Autodesk Inventor part; units mm, degrees
ref_plane "YZ Plane" through (0, 0, 0) normal (1, 0, 0) x (0, 1, 0)
ref_plane "XZ Plane" through (0, 0, 0) normal (0, 1, 0) x (-1, 0, 0)
ref_plane "XY Plane" through (0, 0, 0) normal (0, 0, 1) x (1, 0, 0)
sketch "Sketch1" plane through (0, 0, 0) normal (0, 0, 1) x (1, 0, 0)
  circle A0 centre (0, 0) radius 3.175
  circle A1 centre (0, 0) radius 3.9688
  dimension "d0" = 6.35
  dimension "d1" = 7.9375
extrude "Extrusion1" add sketch "Sketch1" along normal blind 1.8415 contours A0 | A1
extrude "Extrusion2" add sketch "Sketch1" against normal blind 6.35 contours A0
sketch "Sketch2" plane through (0, 0, 1.8415) normal (0, 0, 1) x (1, 0, 0)
  circle A0 centre (0, 0) radius 3.9687
  circle A1 centre (0, 0) radius 3.175
  dimension "d6" = 6.35
extrude "Extrusion3" add sketch "Sketch2" along normal blind 9.525 contours A1
properties part number "Encoder Idler Shaft"
Geometry check sheet. Reference: the model listing, model coordinates, mm. A direction names the side the tool comes from. Give positions to 0.01 mm unless a question says otherwise; leave off trailing zeros. Loops run counter-clockwise (first coordinate to the right, second up) from the corner with the lowest first, then second, coordinate; pieces in that order, holes last.
(1) Set-up check for faces 1 (the flat face through (0, 0, 11.366)), 2 (the cylindrical face through (-0.69, -3.1, -3.13)), 3 (the flat face through (-2, 3, 1.842)): record each of +Z, -Z, +X, -X, +Y, -Y from which the full face is reachable in a straight line by a thin tool's end or side.
From the geometry:
face 1: +Z, +X, -X, +Y, -Y
face 2: -Z
face 3: +Z
(2) Thickness scan on L1, parallel to Z at x = -1.5, y = -3.25; L2, parallel to Y at x = 2.5, z = 4; L3, parallel to X at y = 0.25, z = 8.75. Record the ranges inside material, lowest first.
From the geometry:
L1: z = 0 to 1.84
L2: y = -1.96 to 1.96
L3: x = -3.17 to 3.17
(3) Section check D-D on x = -3.5. Record the cut outline in (y, z), then the cut area to 3 significant figures.
From the geometry:
outline: (-1.87, 0) - (1.87, 0) - (1.87, 1.84) - (-1.87, 1.84) - close
area: 6.89 mm2
(4) Section check C-C on z = 4. Record the cut outline in (x, y) (3 decimals), then the cut area to 3 significant figures.
From the geometry:
outline: circle Ø6.35 at (0, 0)
area: 31.7 mm2
(5) Depth check by flat-ended pin: pin 1 Ø4 at (x, z) = (-1, -1.5) entering from -Y; pin 2 Ø2 at (y, z) = (1.5, 1.5) entering from -X; pin 3 Ø1.5 at (x, z) = (-2, 8) entering from +Y. Enter the tip coordinate at first touch or a pass-through.
From the geometry:
pin 1: stops at y = -3.97
pin 2: stops at x = -3.94
pin 3: stops at y = 2.92
